Here's the drawing with two shaded views (mm, measured from the low corner). I have some questions. A direction names the side the tool comes from. Round coordinates to 2 decimals unless told otherwise and drop trailing zeros. Loops run counter-clockwise (first coordinate to the right, second up) from the corner with the lowest first, then second, coordinate; pieces in that order, holes last. Notation, with made-up numbers: (-1, 20.25) -> (4, 20.25) arc R21 ccw to (4, 58.25) -> close; hole circle Ø2 at (80, 80). An arc over 180 degrees is marked (long way). Write each question's results on one line, items separated by ' | '.
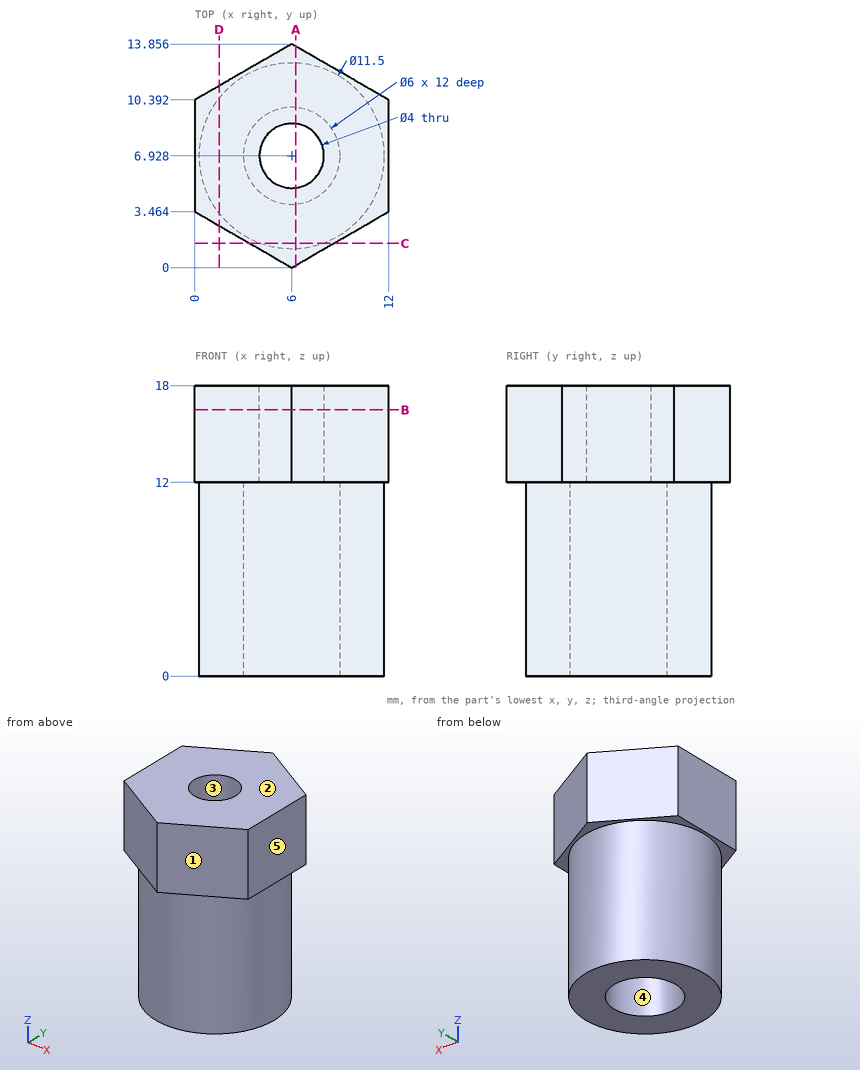
1. If we section it at D-D (x = 1.5): List the corners of the cut face in (y, z) for me, then the cut area to 3 significant figures.
Final values:
outline: (2.6, 12) -> (3.35, 12) -> (3.35, 0) -> (10.51, 0) -> (10.51, 12) -> (11.26, 12) -> (11.26, 18) -> (2.6, 18) -> close | area: 138 mm2
2. On a 3-axis mill with a long thin cutter (end or side, diameter ignored), from which of +Z, -Z, +X, -X, +Y, -Y can I reach the whole of each face in a straight line? I mean the marked faces 4 and 5. Say none if no direction works.
Final values:
face 4: -Z | face 5: +Z, -Z, +X, +Y, -Y
3. If we section it at A-A (x = 6.25): List the corners of the cut face in (y, z) for me (1 decimal).
Final values:
outline: (0.1, 12) -> (1.2, 12) -> (1.2, 0) -> (3.9, 0) -> (3.9, 12) -> (4.9, 12) -> (4.9, 18) -> (0.1, 18) -> close; (8.9, 12) -> (9.9, 12) -> (9.9, 0) -> (12.7, 0) -> (12.7, 12) -> (13.7, 12) -> (13.7, 18) -> (8.9, 18) -> close
4. We'd pull the mould along Y, two halves only. Please class the marked faces 1, 2 and 3: pulls with the +Y half, pulls with the -Y half, needs draft (parallel to the pull), parting line crosses it, or undercut.
Final values:
face 1: pulls with the -Y half | face 2: needs draft | face 3: undercut
5. Please list where these lines run through material, in increasing order: line 1 (Y direction, x = 5.5, z = 17.5) (1 decimal); line 2 (Y direction, x = 6.75, z = 4.25); line 3 (Z direction, x = 7, y = 9.25). Write a range as from..to.
Final values:
line 1: 0.3..5, 8.9..13.6 | line 2: 1.23..4.02, 9.83..12.63 | line 3: 12..18
6. If we section it at B-B (z = 16.5): List the corners of the cut face in (x, y) for me, then the cut area to 3 significant figures.
Final values:
outline: (0, 3.46) -> (6, 0) -> (12, 3.46) -> (12, 10.39) -> (6, 13.86) -> (0, 10.39) -> close; hole circle Ø4 at (6, 6.93) | area: 112 mm2
7. If we section it at C-C (y = 1.5): List the corners of the cut face in (x, z) for me.
Final values:
outline: (3.4, 12) -> (4.1, 12) -> (4.1, 0) -> (7.9, 0) -> (7.9, 12) -> (8.6, 12) -> (8.6, 18) -> (3.4, 18) -> close
8. Will these pins go through, and if not, where does the flat tip stop? pin 1 (5.5 mm diameter, centred on x = 6, y = 6.93, fed in from -Z); pin 2 (5 mm diameter, centred on x = 3.5, z = 11, fed in from +Y) (1 decimal); pin 3 (1.5 mm diameter, centred on x = 6, z = 3, fed in from -Y).
Final values:
pin 1: z = 12 | pin 2: y = 13.7 | pin 3: y = 1.18
